from build123d import *

# Parameters (mm, degrees)
F1_DEPTH = 70
F2_START = -15
F0_R     = 1
F2_DEPTH = 5
F3_START = -55
F3_DEPTH = 5


with BuildPart() as f1:
    # F0 (on Front) → F1 (new body)
    with BuildSketch(Plane.XZ):
        with BuildLine():
            Line((81.2036521524, 41.5010131064), (-86.0963478476, 41.5010131064))
            ThreePointArc((-86.0963478476, 41.5010131064), (-90.5864759081, 39.6411411669), (-92.4463478476, 35.1510131064))
            Line((-92.4463478476, 35.1510131064), (-92.4463478476, -22.1489868936))
            ThreePointArc((-92.4463478476, -22.1489868936), (-90.5864759081, -26.6391149541), (-86.0963478476, -28.4989868936))
            Line((-86.0963478476, -28.4989868936), (81.2036521524, -28.4989868936))
            ThreePointArc((81.2036521524, -28.4989868936), (85.693780213, -26.6391149541), (87.5536521524, -22.1489868936))
            Line((87.5536521524, -22.1489868936), (87.5536521524, 35.1510131064))
            ThreePointArc((87.5536521524, 35.1510131064), (85.693780213, 39.6411411669), (81.2036521524, 41.5010131064))
        make_face()
        Polygon((-87.4463478476, 16.5010131064), (-87.4463478476, 36.5010131064), (-67.4463478476, 36.5010131064), (-62.4463478476, 36.5010131064), (-7.4463478476, 36.5010131064), (62.5536521524, 36.5010131064), (82.5536521524, 36.5010131064), (82.5536521524, 16.5010131064), (82.5536521524, -3.4989868936), (82.5536521524, -23.4989868936), (62.5536521524, -23.4989868936), (-7.4463478476, -23.4989868936), (-12.4463478476, -23.4989868936), (-62.4463478476, -23.4989868936), (-67.4463478476, -23.4989868936), (-87.4463478476, -23.4989868936), (-87.4463478476, -3.4989868936), align=None, mode=Mode.SUBTRACT)
    extrude(amount=-F1_DEPTH)

    # F0 (on Front) → F2 (join)
    with BuildSketch(Plane.XZ.offset(F2_START)):
        with BuildLine():
            Line((-73.7963478476, -3.4989868936), (-87.4463478476, -3.4989868936))
            Line((-87.4463478476, -3.4989868936), (-87.4463478476, -23.4989868936))
            Line((-87.4463478476, -23.4989868936), (-67.4463478476, -23.4989868936))
            Line((-67.4463478476, -23.4989868936), (-67.4463478476, -18.4989868936))
            Line((-67.4463478476, -18.4989868936), (-67.4463478476, -9.8489868936))
            ThreePointArc((-67.4463478476, -9.8489868936), (-69.306219787, -5.3588588331), (-73.7963478476, -3.4989868936))
        make_face()
        with Locations((-77.4463478476, -13.4989868936)):
            Circle(F0_R, mode=Mode.SUBTRACT)
        with BuildLine():
            Line((62.5536521524, -9.8489868936), (62.5536521524, -23.4989868936))
            Line((62.5536521524, -23.4989868936), (82.5536521524, -23.4989868936))
            Line((82.5536521524, -23.4989868936), (82.5536521524, -3.4989868936))
            Line((82.5536521524, -3.4989868936), (68.9036521524, -3.4989868936))
            ThreePointArc((68.9036521524, -3.4989868936), (64.4135240919, -5.3588588331), (62.5536521524, -9.8489868936))
        make_face()
        with Locations((72.5536521524, -13.4989868936)):
            Circle(F0_R, mode=Mode.SUBTRACT)
        with BuildLine():
            Line((82.5536521524, 36.5010131064), (62.5536521524, 36.5010131064))
            Line((62.5536521524, 36.5010131064), (62.5536521524, 22.8510131064))
            ThreePointArc((62.5536521524, 22.8510131064), (64.4135240919, 18.3608850459), (68.9036521524, 16.5010131064))
            Line((68.9036521524, 16.5010131064), (82.5536521524, 16.5010131064))
            Line((82.5536521524, 16.5010131064), (82.5536521524, 36.5010131064))
        make_face()
        with Locations((72.5536521524, 26.5010131064)):
            Circle(F0_R, mode=Mode.SUBTRACT)
        with BuildLine():
            Line((-67.4463478476, 36.5010131064), (-87.4463478476, 36.5010131064))
            Line((-87.4463478476, 36.5010131064), (-87.4463478476, 16.5010131064))
            Line((-87.4463478476, 16.5010131064), (-73.7963478476, 16.5010131064))
            ThreePointArc((-73.7963478476, 16.5010131064), (-69.306219787, 18.3608850459), (-67.4463478476, 22.8510131064))
            Line((-67.4463478476, 22.8510131064), (-67.4463478476, 36.5010131064))
        make_face()
        with Locations((-77.4463478476, 26.5010131064)):
            Circle(F0_R, mode=Mode.SUBTRACT)
    extrude(amount=-F2_DEPTH)

    # F0 (on Front) → F3 (join)
    with BuildSketch(Plane.XZ.offset(F3_START)):
        with BuildLine():
            Line((82.5536521524, 36.5010131064), (62.5536521524, 36.5010131064))
            Line((62.5536521524, 36.5010131064), (62.5536521524, 22.8510131064))
            ThreePointArc((62.5536521524, 22.8510131064), (64.4135240919, 18.3608850459), (68.9036521524, 16.5010131064))
            Line((68.9036521524, 16.5010131064), (82.5536521524, 16.5010131064))
            Line((82.5536521524, 16.5010131064), (82.5536521524, 36.5010131064))
        make_face()
        with Locations((72.5536521524, 26.5010131064)):
            Circle(F0_R, mode=Mode.SUBTRACT)
        with BuildLine():
            Line((62.5536521524, -9.8489868936), (62.5536521524, -23.4989868936))
            Line((62.5536521524, -23.4989868936), (82.5536521524, -23.4989868936))
            Line((82.5536521524, -23.4989868936), (82.5536521524, -3.4989868936))
            Line((82.5536521524, -3.4989868936), (68.9036521524, -3.4989868936))
            ThreePointArc((68.9036521524, -3.4989868936), (64.4135240919, -5.3588588331), (62.5536521524, -9.8489868936))
        make_face()
        with Locations((72.5536521524, -13.4989868936)):
            Circle(F0_R, mode=Mode.SUBTRACT)
        with BuildLine():
            Line((-73.7963478476, -3.4989868936), (-87.4463478476, -3.4989868936))
            Line((-87.4463478476, -3.4989868936), (-87.4463478476, -23.4989868936))
            Line((-87.4463478476, -23.4989868936), (-67.4463478476, -23.4989868936))
            Line((-67.4463478476, -23.4989868936), (-67.4463478476, -18.4989868936))
            Line((-67.4463478476, -18.4989868936), (-67.4463478476, -9.8489868936))
            ThreePointArc((-67.4463478476, -9.8489868936), (-69.306219787, -5.3588588331), (-73.7963478476, -3.4989868936))
        make_face()
        with Locations((-77.4463478476, -13.4989868936)):
            Circle(F0_R, mode=Mode.SUBTRACT)
        with BuildLine():
            Line((-67.4463478476, 36.5010131064), (-87.4463478476, 36.5010131064))
            Line((-87.4463478476, 36.5010131064), (-87.4463478476, 16.5010131064))
            Line((-87.4463478476, 16.5010131064), (-73.7963478476, 16.5010131064))
            ThreePointArc((-73.7963478476, 16.5010131064), (-69.306219787, 18.3608850459), (-67.4463478476, 22.8510131064))
            Line((-67.4463478476, 22.8510131064), (-67.4463478476, 36.5010131064))
        make_face()
        with Locations((-77.4463478476, 26.5010131064)):
            Circle(F0_R, mode=Mode.SUBTRACT)
    extrude(amount=-F3_DEPTH)


solid = f1.part
Could you check a few things on this model? Use its own coordinates, in mm. A direction names the side the tool comes from. Coordinates: 2 decimals unless noted, no trailing zeros. Loops run counter-clockwise (first coordinate to the right, second up) from the corner with the lowest first, then second, coordinate; pieces in that order, holes last.
1. I need wall thicknesses on L1, parallel to Z at x = -62.5, y = 25; L2, parallel to X at y = 65, z = 8.5; L3, parallel to Y at x = 75, z = -15. Which ranges of each line are inside material? Lowest first, please.
2. Imagine slicing it at C-C (y = 38.5). Please give me the cut outline in (x, z), and give its area (3 significant figures).
3. Imagine slicing it at D-D (z = 12). Please give me the cut outline in (x, y), and give its area (3 significant figures).
4. Imagine slicing it at A-A (z = -20). Please give me the cut outline in (x, y), and give its area (3 significant figures).
5. Imagine slicing it at B-B (x = -20). Please give me the cut outline in (y, z), and give its area (3 significant figures).
6. For P1, Ø22, axis at x = -81.5, z = -10.5, coming from the +Y side; P2, Ø6, axis at x = -75.5, z = -17.5, coming from the -Y side; P3, Ø6, axis at x = -74, z = 25, coming from the +Y side, each with a flat end and sliding along its axis, tell me the tip position at first contact or that it passes through.
7. For faces 1 (the face through (-78, 15, 29)), 2 (the face through (76, 57, 16.501)), 3 (the face through (-78, 60, -16)), 4 (the face through (-78, 20, 29)), 5 (the face through (-10, 70, -24)), which set-ups out of +Z, -Z, +X, -X, +Y, -Y let a thin tool reach every point of the face, with its end or its side?
8. We'd pull the mould along X, two halves only. Please class faces 6 (the face through (-78, 55, 29)), 7 (the face through (85.743, 34.51, 39.591)), 8 (the face through (-90.537, 34.51, 39.69)): released by +X, released by -X, zero draft, split by the parting line, or undercut.
Computed values:
1. L1: z = -28.5 to -23.5, 36.5 to 41.5
1. L2: x = -92.45 to -87.45, 82.55 to 87.55
1. L3: y = 15 to 20, 55 to 60
2. outline: (-92.45, -22.15) arc R6.35 ccw to (-86.1, -28.5) - (81.2, -28.5) arc R6.35 ccw to (87.55, -22.15) - (87.55, 35.15) arc R6.35 ccw to (81.2, 41.5) - (-86.1, 41.5) arc R6.35 ccw to (-92.45, 35.15) - close; hole (-87.45, -23.5) - (82.55, -23.5) - (82.55, 36.5) - (-87.45, 36.5) - close
2. area: 2,370 mm2
3. outline: (-92.45, 0) - (-87.45, 0) - (-87.45, 70) - (-92.45, 70) - close; (82.55, 0) - (87.55, 0) - (87.55, 70) - (82.55, 70) - close
3. area: 700 mm2
4. outline: (-92.45, 0) - (-87.45, 0) - (-87.45, 15) - (-67.45, 15) - (-67.45, 20) - (-87.45, 20) - (-87.45, 55) - (-67.45, 55) - (-67.45, 60) - (-87.45, 60) - (-87.45, 70) - (-92.45, 70) - close; (62.55, 15) - (82.55, 15) - (82.55, 0) - (87.55, 0) - (87.55, 70) - (82.55, 70) - (82.55, 60) - (62.55, 60) - (62.55, 55) - (82.55, 55) - (82.55, 20) - (62.55, 20) - close
4. area: 1,100 mm2
5. outline: (0, -28.5) - (70, -28.5) - (70, -23.5) - (0, -23.5) - close; (0, 36.5) - (70, 36.5) - (70, 41.5) - (0, 41.5) - close
5. area: 700 mm2
6. P1: stops at y = 70
6. P2: stops at y = 15
6. P3: stops at y = 60
7. face 1: -Y
7. face 2: +Y, -Y
7. face 3: +Y
7. face 4: none
7. face 5: +Z, -Z, +X, -X, +Y
8. face 6: undercut
8. face 7: released by +X
8. face 8: released by -X
